Autodesk Inventor part; units mm, degrees
ref_plane "YZ Plane" through (0, 0, 0) normal (1, 0, 0) x (0, 1, 0)
ref_plane "XZ Plane" through (0, 0, 0) normal (0, 1, 0) x (-1, 0, 0)
ref_plane "XY Plane" through (0, 0, 0) normal (0, 0, 1) x (1, 0, 0)
sketch "Sketch_1" plane through (0, 0, 0) normal (0, 0, 1) x (1, 0, 0)
  line L0 (6, 0) -> (0, 0)
  line L1 (-0.8, 0) -> (-0.8, 2.7673)
  line L2 (-0.8, 2.7673) -> (-0.5333, 3.5)
  line L3 (-0.5333, 3.5) -> (0, 3.5)
  line L4 (0, 3.5) -> (0, 1.9)
  arc A0 (0, 1.9) -> (0.4, 1.5) centre (0.4, 1.9) ccw
  line L5 (0.4, 1.5) -> (6, 1.5)
  line L6 (6, 1.5) -> (6, 0)
  line L7 (6, 0) -> (-0.8, 0)
  line L8 (0, 0) -> (-0.8, 0)
  dimension "d6" = 6
revolve "Revolution1" add sketch "Sketch_1" angle 360 about axis through (6, 0, 0) along (1, 0, 0)
sketch "Sketch_5" plane through (-0.05, 0, 0) normal (1, 0, 0) x (0, 0, -1)
  arc A0 (-0.6801, -0.1159) -> (-0.4404, -0.531) centre (-0.5499, -0.3175) ccw
  arc A1 (-0.341, -0.5357) -> (-0.4404, -0.531) centre (-0.3947, -0.62) ccw
  arc A2 (-0.341, -0.5357) -> (-0.2934, -0.5632) centre (0, 0) ccw
  arc A3 (-0.2397, -0.6469) -> (-0.2934, -0.5632) centre (-0.3396, -0.6519) ccw
  arc A4 (-0.2397, -0.6469) -> (0.2397, -0.6469) centre (0, -0.635) ccw
  arc A5 (0.2934, -0.5632) -> (0.2397, -0.6469) centre (0.3396, -0.6519) ccw
  arc A6 (0.2934, -0.5632) -> (0.341, -0.5357) centre (0, 0) ccw
  arc A7 (0.4404, -0.531) -> (0.341, -0.5357) centre (0.3947, -0.62) ccw
  arc A8 (0.4404, -0.531) -> (0.6801, -0.1159) centre (0.5499, -0.3175) ccw
  arc A9 (0.6344, -0.0275) -> (0.6801, -0.1159) centre (0.7343, -0.0318) ccw
  arc A10 (0.6344, -0.0275) -> (0.6344, 0.0275) centre (0, 0) ccw
  arc A11 (0.6801, 0.1159) -> (0.6344, 0.0275) centre (0.7343, 0.0318) ccw
  arc A12 (0.6801, 0.1159) -> (0.4404, 0.531) centre (0.5499, 0.3175) ccw
  arc A13 (0.341, 0.5357) -> (0.4404, 0.531) centre (0.3947, 0.62) ccw
  arc A14 (0.341, 0.5357) -> (0.2934, 0.5632) centre (0, 0) ccw
  arc A15 (0.2397, 0.6469) -> (0.2934, 0.5632) centre (0.3396, 0.6519) ccw
  arc A16 (0.2397, 0.6469) -> (-0.2397, 0.6469) centre (0, 0.635) ccw
  arc A17 (-0.2934, 0.5632) -> (-0.2397, 0.6469) centre (-0.3396, 0.6519) ccw
  arc A18 (-0.2934, 0.5632) -> (-0.341, 0.5357) centre (0, 0) ccw
  arc A19 (-0.4404, 0.531) -> (-0.341, 0.5357) centre (-0.3947, 0.62) ccw
  arc A20 (-0.4404, 0.531) -> (-0.6801, 0.1159) centre (-0.5499, 0.3175) ccw
  arc A21 (-0.6344, 0.0275) -> (-0.6801, 0.1159) centre (-0.7343, 0.0318) ccw
  arc A22 (-0.6344, 0.0275) -> (-0.6344, -0.0275) centre (0, 0) ccw
  arc A23 (-0.6801, -0.1159) -> (-0.6344, -0.0275) centre (-0.7343, -0.0318) ccw
extrude "Extrusion1" cut sketch "Sketch_5" against normal blind 0.75
sketch "Sketch_2" plane through (0, 0, 0) normal (0, 0, 1) x (1, 0, 0)
  line L0 (0.4552, 0) -> (0, 0)
  line L1 (-0.05, 0) -> (-0.05, 0.875)
  line L2 (-0.05, 0.875) -> (0.4552, 0)
  line L3 (0.4552, 0) -> (-0.05, 0)
revolve "Revolution2" cut sketch "Sketch_2" angle 360 about axis through (0.4552, 0, 0) along (1, 0, 0)
sketch "スケッチ4" plane through (6, 0, 0) normal (1, 0, 0) x (0, 0, -1)
  circle A0 centre (0, 0) radius 1.5
extrude "押し出し2" add sketch "スケッチ4" along normal blind 2
thread "Thread1"
properties part number "超極低頭ネジL8" material "ステンレス鋼"
The model under review builds one solid part; all positions refer to its coordinate system, in mm. A direction names the side the tool comes from. Give positions to 0.01 mm unless a question says otherwise; leave off trailing zeros. Write each loop counter-clockwise with the first axis right and the second up, starting at its lowest first coordinate (ties: lowest second). Pieces come first, ordered by that corner, then holes.
1. Draft analysis for pull direction Y (two halves, no side actions). For faces 3 (the conical face through (0.367, -0.033, 0.148)), 4 (the flat face through (8, 0, 0)), 5 (the cylindrical face through (-0.263, 3.233, -1.341)), state which applies: +Y half, -Y half, draft (parallel to the pull), parting line (faces both ways), or undercut.
2. For P1, Ø1.5, axis at y = -2, z = -3, coming from the +X side; P2, Ø1.5, axis at x = 6.5, z = 2, coming from the -Y side, all flat-tipped, find the tip position at first contact; note any pin that passes through.
3. Tool access review of faces 1 (the flat face through (0, 2, -2)), 2 (the flat face through (-0.8, 0, 1)): name each direction out of +Z, -Z, +X, -X, +Y, -Y from which nothing blocks a thin tool from reaching the whole face with its end or side.
4. Add section A-A, the plane x = 4. Write out the cut boundary in (y, z).
5. Wall thickness on L1, parallel to X at y = 2.25, z = -1; L2, parallel to Z at x = 3.75, y = 0; L3, parallel to X at y = 0.75, z = 3: over which ranges is each line inside the solid? List them lowest first.
Worked answers:
1. face 3: undercut
1. face 4: draft
1. face 5: parting line
2. P1: stops at x = 0
2. P2: stops at y = -0.83
3. face 1: +X
3. face 2: +Z, -Z, -X, +Y, -Y
4. outline: circle Ø3 at (0, 0)
5. L1: x = -0.8 to 0
5. L2: z = -1.5 to 1.5
5. L3: x = -0.68 to 0
